Can you work these out from the model? Positions are in its coordinate system, mm. Coordinates: 2 decimals unless noted, no trailing zeros. Order: outer loops, then holes, each group sorted by start corner. A loop starts at its lowest first (then second) coordinate and runs counter-clockwise, first axis right, second up. Notation, with made-up numbers: (-14.75, 69.5) -> (16.25, 69.5) arc R14 ccw to (16.25, 96.5) -> close; hole circle Ø7 at (69, 5). An arc over 180 degrees is marked (long way). Write item = value, one per line.
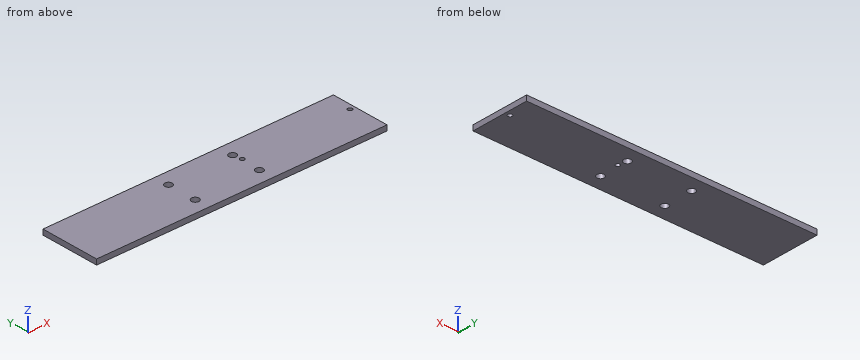
Autodesk Inventor part; units mm, degrees
ref_plane "YZ Plane" through (0, 0, 0) normal (1, 0, 0) x (0, 1, 0)
ref_plane "XZ Plane" through (0, 0, 0) normal (0, 1, 0) x (-1, 0, 0)
ref_plane "XY Plane" through (0, 0, 0) normal (0, 0, 1) x (1, 0, 0)
sketch "Sketch1" plane through (0, 0, 0) normal (0, 0, 1) x (1, 0, 0)
  line L0 (0, 0) -> (175.26, 0)
  line L1 (175.26, 0) -> (175.26, -35.56)
  line L2 (175.26, -35.56) -> (0, -35.56)
  line L3 (0, -35.56) -> (0, 0)
  dimension "d0" = 175.26
  dimension "d1" = 35.56
extrude "Extrusion1" add sketch "Sketch1" along normal blind 3.175
sketch "Sketch7" plane through (0, 0, 3.175) normal (0, 0, 1) x (1, 0, 0)
  line L0 (0, 0) -> (175.26, 0)
  line L1 (175.26, -35.56) -> (0, -35.56)
  line L2 (111.125, 1.27) -> (111.125, -35.56)
  line L3 (111.125, 1.27) -> (101.6, 1.27)
  line L4 (101.6, -35.56) -> (101.6, 1.27)
  line L5 (111.125, -35.56) -> (101.6, -35.56)
  line L6 (62.865, 1.27) -> (62.865, -35.56)
  line L7 (62.865, -35.56) -> (72.39, -35.56)
  line L8 (72.39, -35.56) -> (72.39, 1.27)
  line L9 (62.865, 1.27) -> (72.39, 1.27)
  circle A0 centre (106.3625, -26.67) radius 1.651
  circle A1 centre (106.3625, -8.89) radius 1.651
  point P0 (67.6275, -8.89)
  point P1 (67.6275, -26.67)
  point P2 (106.3625, -8.89)
  point P3 (106.3625, -26.67)
  dimension "d97" = 26.67
  dimension "d98" = 8.89
  dimension "d99" = 8.89
  dimension "d100" = 26.67
  dimension "d101" = 8.89
hole "Hole5" at (67.6275, -8.89, 3.175) at (67.6275, -26.67, 3.175) at (106.3625, -8.89, 3.175) at (106.3625, -26.67, 3.175) direction (0, 0, -1) diameter 4.4958 end through all
sketch "Sketch8" plane through (0, 0, 3.175) normal (0, 0, 1) x (1, 0, 0)
  arc A0 (172.26, -12.306) -> (172.26, -16.306) centre (172.26, -14.306) ccw
  arc A1 (107.26, -16.306) -> (107.26, -12.306) centre (107.26, -14.306) ccw
hole "Hole6" at (107.26, -14.306, 3.175) at (172.26, -14.306, 3.175) direction (0, 0, -1) diameter 2.6416 end through all
properties part number "Battery Board" material "Aluminum-6061"
Item 1: I want a section at A-A, the plane y = -8.89. Please give me the cut outline in (x, z) (3 decimals).
A:
outline = (0, 0) -> (65.38, 0) -> (65.38, 3.175) -> (0, 3.175) -> close; (69.875, 0) -> (104.115, 0) -> (104.115, 3.175) -> (69.875, 3.175) -> close; (108.61, 0) -> (175.26, 0) -> (175.26, 3.175) -> (108.61, 3.175) -> close
Item 2: I'm going to push a flat-ended pin straight in: P1, Ø3, axis at x = 172.26, y = -14.306, coming from the -Z side. Where does the tip first touch, or does it pass through?
A:
P1 = 0
Item 3: If I drill on probe 1 along X at (y, z) = (-14, 0.25); probe 2 along X at (y, z) = (-9, 2.95); probe 3 along Y at (x, z) = (66.5, 2.4), over which ranges is the centre line in solid material (lowest first)?
A:
probe_1 = 0 to 105.98, 108.54 to 170.98, 173.54 to 175.26
probe_2 = 0 to 65.38, 69.87 to 104.12, 108.61 to 175.26
probe_3 = -35.56 to -28.61, -24.73 to -10.83, -6.95 to 0
